Check sheet for the modelled part. Datum: model origin and axes. Units: mm. A direction names the side the tool comes from. Round coordinates to 2 decimals unless told otherwise and drop trailing zeros. Loops run counter-clockwise (first coordinate to the right, second up) from the corner with the lowest first, then second, coordinate; pieces in that order, holes last. Notation, with made-up numbers: (38.25, 72) - (56.25, 72) arc R11 ccw to (56.25, 83) - close; hole circle Ø9 at (-17.5, 68.5). An arc over 180 degrees is marked (long way). Return JSON: item names as keys, results as strings.
from build123d import *

# Parameters (mm, degrees)
SKETCH_1_R          = 2.05
SKETCH_1_R_2        = 2.5
SKETCH_1_R_3        = 3
SKETCH_1_R_4        = 1.6
EXTRUDE_1_DEPTH     = 5
SKETCH_2_R          = 2.25
CUT_EXTRUDE_1_DEPTH = 1.5


with BuildPart() as part:
    # 草图1 → 凸台-拉伸1 (new body)
    with BuildSketch(Plane(origin=(0, 0, 0), x_dir=(0, 0, -1), z_dir=(1, 0, 0))):
        with BuildLine():
            Line((5, 0), (5, 55.679491924))
            ThreePointArc((5, 55.679491924), (4.330127019, 58.179491924), (2.5, 60.009618943))
            Line((2.5, 60.009618943), (-27.5, 77.330127019))
            ThreePointArc((-27.5, 77.330127019), (-34.095760221, 75.867882182), (-33.213938048, 69.169777784))
            Line((-33.213938048, 69.169777784), (-12.144247806, 51.490208473))
            ThreePointArc((-12.144247806, 51.490208473), (-6.873844259, 44.621684846), (-5, 36.169319611))
            Line((-5, 36.169319611), (-5, 0))
            ThreePointArc((-5, 0), (0, -5), (5, 0))
        make_face()
        Circle(SKETCH_1_R, mode=Mode.SUBTRACT)
        with Locations((0, 20)):
            Circle(SKETCH_1_R_2, mode=Mode.SUBTRACT)
        with Locations((0, 55)):
            Circle(SKETCH_1_R_3, mode=Mode.SUBTRACT)
        with Locations((-30, 73)):
            Circle(SKETCH_1_R_4, mode=Mode.SUBTRACT)
    extrude(amount=EXTRUDE_1_DEPTH)

    # 草图2 → 切除-拉伸1 (cut)
    with BuildSketch(Plane.ZY):
        with Locations((30, 73)):
            Circle(SKETCH_2_R)
    extrude(amount=-CUT_EXTRUDE_1_DEPTH, mode=Mode.SUBTRACT)


solid = part.part
Q1. Depth check by flat-ended pin: P1, Ø4, axis at y = 73, z = 30, coming from the -X side; P2, Ø2.5, axis at x = 2, y = 26.5, coming from the +Z side. Enter the tip coordinate at first touch or a pass-through.
Answer key:
{"P1": "stops at x = 1.5", "P2": "stops at z = 5"}
Q2. Draft check along Y on faces 1 (the face through (2, 76, 34)), 2 (the face through (2.465, 44.732, 6.926)), 3 (the face through (5, 43, 5)), 4 (the face through (2.46, 22.48, 0.33)). Enter one of: released by +Y, released by -Y, zero draft, split by the parting line, or undercut.
Answer key:
{"face 1": "split by the parting line", "face 2": "released by -Y", "face 3": "zero draft", "face 4": "undercut"}
Q3. Scan lines: probe 1 along Y at (x, z) = (1.65, 0); probe 2 along Y at (x, z) = (2.2, 1); probe 3 along Z at (x, y) = (1.2, 22). Record each from-to range of solid material in increasing order. Write a range as [from, to].
Answer key:
{"probe 1": "y = [-5, -2.05], [2.05, 17.5], [22.5, 52], [58, 61.45]", "probe 2": "y = [-4.9, -1.79], [1.79, 17.71], [22.29, 52.17], [57.83, 62.03]", "probe 3": "z = [-5, -1.5], [1.5, 5]"}
Q4. Tool access check on faces 5 (the face through (2.465, 2.033, 0.267)), 6 (the face through (0.74, 70.804, 29.512)), 7 (the face through (2, 18, 5)). Record the directions out of +Z, -Z, +X, -X, +Y, -Y that give a thin tool (end or side, any length) a straight path to the whole face; none if there is none.
Answer key:
{"face 5": "+X, -X", "face 6": "-X", "face 7": "+Z, +X, -X, -Y"}
Q5. Sectioned sample at A-A (y = 73). Enter the section's corners in (x, z), plus the area to 4 significant figures.
Answer key:
{"outline": "(0, 20) - (5, 20) - (5, 28.4) - (1.5, 28.4) - (1.5, 27.75) - (0, 27.75) - close; (0, 32.25) - (1.5, 32.25) - (1.5, 31.6) - (5, 31.6) - (5, 35) - (0, 35) - close", "area": "57.05 mm²"}
Q6. Sectioned sample at D-D (z = 9). Enter the section's corners in (x, y), plus the area to 3 significant figures.
Answer key:
{"outline": "(0, 48.17) - (5, 48.17) - (5, 66.65) - (0, 66.65) - close", "area": "92.4 mm²"}
Q7. Sectioned sample at C-C (z = 30). Enter the section's corners in (x, y), plus the area to 3 significant figures.
Answer key:
{"outline": "(0, 66.47) - (5, 66.47) - (5, 71.4) - (1.5, 71.4) - (1.5, 70.75) - (0, 70.75) - close; (0, 75.25) - (1.5, 75.25) - (1.5, 74.6) - (5, 74.6) - (5, 78) - (0, 78) - close", "area": "39.7 mm²"}
Q8. Sectioned sample at B-B (x = 2.5). Enter the section's corners in (y, z).
Answer key:
{"outline": "(0, -5) - (55.68, -5) arc R5 ccw to (60.01, -2.5) - (77.33, 27.5) arc R5 ccw to (69.17, 33.21) - (51.49, 12.14) arc R20 cw to (36.17, 5) - (0, 5) arc R5 ccw to start; hole circle Ø4.1 at (0, 0); hole circle Ø5 at (20, 0); hole circle Ø6 at (55, 0); hole circle Ø3.2 at (73, 30)"}
